```python
from build123d import *

# Parameters (mm, degrees)
F0_W     = 50.8
F0_H     = 25.4
F1_DEPTH = 25.4
F2_R     = 3.81
F3_DEPTH = 63.5
F6_SIZE  = 5.08


with BuildPart() as f1:
    # F0 (on Top) → F1 (new body)
    with BuildSketch(Plane.XY):
        Rectangle(F0_W, F0_H)
    extrude(amount=F1_DEPTH)

    # F2 (on face) → F3 (join)
    with BuildSketch(Plane.XY.offset(25.4)):
        Circle(F2_R)
    extrude(amount=F3_DEPTH)

    # F4 (on face) → F5 (revolve)
    with BuildSketch(Plane.XY.offset(88.9)):
        with BuildLine():
            Line((0, 3.81), (0, -3.81))
            ThreePointArc((0, -3.81), (2.694077, -2.694077), (3.81, 0))
            ThreePointArc((3.81, 0), (2.694077, 2.694077), (0, 3.81))
        make_face()
    revolve(axis=Axis((0, 0, 88.9), (0, -1, 0)))

    # F6
    f6_edges = [f1.edges().sort_by_distance(p)[0] for p in [
        (-25.4, 0, 25.4),
        (25.4, 0, 25.4),
        (0, -12.7, 25.4),
        (0, 12.7, 25.4),
        (0, -12.7, 0),
        (0, 12.7, 0),
        (-25.4, 0, 0),
        (25.4, 0, 0),
        (25.4, -12.7, 12.7),
        (25.4, 12.7, 12.7),
        (-25.4, 12.7, 12.7),
        (-25.4, -12.7, 12.7),
    ]]
    chamfer(f6_edges, length=F6_SIZE)


solid = f1.part
```
Build history of the part. All positions in model axes, mm. A direction names the side the tool comes from. Round coordinates to 2 decimals unless told otherwise and drop trailing zeros. Order: outer loops, then holes, each group sorted by start corner. A loop starts at its lowest first (then second) coordinate and runs counter-clockwise, first axis right, second up. Notation, with made-up numbers: (28.5, 37) - (52.5, 37) arc R18 cw to (52.5, 42) - close; hole circle Ø7 at (89, 84). An arc over 180 degrees is marked (long way). Use a Markdown table: item, result.
1) Flat gauge pins, fed straight in: pin 1 Ø4 at (x, y) = (-20, -0.5) entering from +Z; pin 2 Ø7.5 at (x, y) = (6.5, -2) entering from +Z; pin 3 Ø4 at (y, z) = (-9.5, 25) entering from +X. Where does each tip first touch, or does it go through?
Recorded:
| item | result |
|---|---|
| pin 1 | stops at z = 25.4 |
| pin 2 | stops at z = 91.18 |
| pin 3 | stops at x = 21.67 |
2) Wall check: L1, parallel to Z at x = -7, y = 3.5; L2, parallel to Z at x = -20.5, y = 7.5; L3, parallel to Y at x = 21, z = 8. Give the ranges that are in metal, low to high.
Recorded:
| item | result |
|---|---|
| L1 | z = 0 to 25.4 |
| L2 | z = 0.18 to 25.22 |
| L3 | y = -12.02 to 12.02 |
3) Tool access for faces 1 (the face through (-22.82, -0.11, 2.5)), 2 (the face through (-0.83, -3.72, 56.71)): list every direction of +Z, -Z, +X, -X, +Y, -Y with a clear straight run to the whole face (end or side of a thin tool).
Recorded:
| item | result |
|---|---|
| face 1 | -Z, -X, +Y, -Y |
| face 2 | +Z |
4) Saw through at B-B on x = -15. Write the cut outline in (y, z), and give its area (3 significant figures).
Recorded:
| item | result |
|---|---|
| outline | (-12.7, 5.08) - (-7.62, 0) - (7.62, 0) - (12.7, 5.08) - (12.7, 20.32) - (7.62, 25.4) - (-7.62, 25.4) - (-12.7, 20.32) - close |
| area | 594 mm² |
5) Saw through at A-A on y = 10. Write the cut outline in (x, z), and give its area (3 significant figures).
Recorded:
| item | result |
|---|---|
| outline | (-23.02, 5.08) - (-20.32, 2.38) - (20.32, 2.38) - (23.02, 5.08) - (23.02, 20.32) - (20.32, 23.02) - (-20.32, 23.02) - (-23.02, 20.32) - close |
| area | 936 mm² |
6) Saw through at C-C on z = 37. Write the cut outline in (x, y), and give its area (3 significant figures).
Recorded:
| item | result |
|---|---|
| outline | circle Ø7.62 at (0, 0) |
| area | 45.6 mm² |
